from build123d import *

# Parameters (mm, degrees)
SKETCH_2_W          = 460
SKETCH_2_H          = 110
EXTRUDE_1_DEPTH     = 8
SKETCH_4_R          = 1.5
CUT_EXTRUDE_1_DEPTH = 237.619948441
SKETCH_3_R          = 2.5
SKETCH_3_R_2        = 1.5
CUT_EXTRUDE_2_DEPTH = 237.619948441
FILLET_1_R          = 10


with BuildPart() as part:
    # 草图2 → 凸台-拉伸1 (new body)
    with BuildSketch(Plane(origin=(0, 0, 0), x_dir=(1, 0, 0), z_dir=(0, 1, 0))):
        Rectangle(SKETCH_2_W, SKETCH_2_H)
    extrude(amount=EXTRUDE_1_DEPTH)

    # 草图4 → 切除-拉伸1 (cut, through all)
    with BuildSketch(Plane(origin=(0, 8, 0), x_dir=(1, 0, 0), z_dir=(0, 1, 0))):
        with Locations(Location((-70, 35, 0), (0, 0, 270))):
            Circle(SKETCH_4_R)
        with Locations(Location((-70, -43, 0), (0, 0, 270))):
            Circle(SKETCH_4_R)
        with Locations(Location((-215, -43, 0), (0, 0, 270))):
            Circle(SKETCH_4_R)
        with Locations(Location((-215, 40, 0), (0, 0, 270))):
            Circle(SKETCH_4_R)
        with Locations(Location((-170, -43, 0), (0, 0, 270))):
            Circle(SKETCH_4_R)
        with Locations(Location((-215, -1.5, 0), (0, 0, 270))):
            Circle(SKETCH_4_R)
    cut_extrude_1 = extrude(amount=-CUT_EXTRUDE_1_DEPTH, mode=Mode.SUBTRACT)

    # 草图3 → 切除-拉伸2 (cut, through all)
    with BuildSketch(Plane(origin=(0, 8, 0), x_dir=(1, 0, 0), z_dir=(0, 1, 0))):
        with Locations(Location((-120, 25, 0), (0, 0, 270))):
            Circle(SKETCH_3_R)
        with Locations(Location((-120, -5, 0), (0, 0, 270))):
            Circle(SKETCH_3_R)
        with Locations(Location((-152, 32.5, 0), (0, 0, 270))):
            Circle(SKETCH_3_R_2)
        with Locations(Location((-152, 22.5, 0), (0, 0, 270))):
            Circle(SKETCH_3_R_2)
        with Locations(Location((-96, 32.5, 0), (0, 0, 270))):
            Circle(SKETCH_3_R_2)
        with Locations(Location((-96, 22.5, 0), (0, 0, 270))):
            Circle(SKETCH_3_R_2)
        Polygon((-70, 55), (-48.5526258, 35), (48.5526258, 35), (70, 55), align=None)
    cut_extrude_2 = extrude(amount=-CUT_EXTRUDE_2_DEPTH, mode=Mode.SUBTRACT)

    # 镜向1: 切除-拉伸1, 切除-拉伸2 across plane
    add(cut_extrude_1.mirror(Plane(origin=(0, 0, 0), x_dir=(0, 0, 1), z_dir=(1, 0, 0))), mode=Mode.SUBTRACT)
    add(cut_extrude_2.mirror(Plane(origin=(0, 0, 0), x_dir=(0, 0, 1), z_dir=(1, 0, 0))), mode=Mode.SUBTRACT)

    # 圆角1
    fillet_1_edges = [part.edges().sort_by_distance(p)[0] for p in [
        (-70, 4, -55),
        (70, 4, -55),
        (48.5526258, 4, -35),
        (-48.5526258, 4, -35),
        (-230, 4, -55),
        (230, 4, -55),
    ]]
    fillet(fillet_1_edges, radius=FILLET_1_R)


solid = part.part
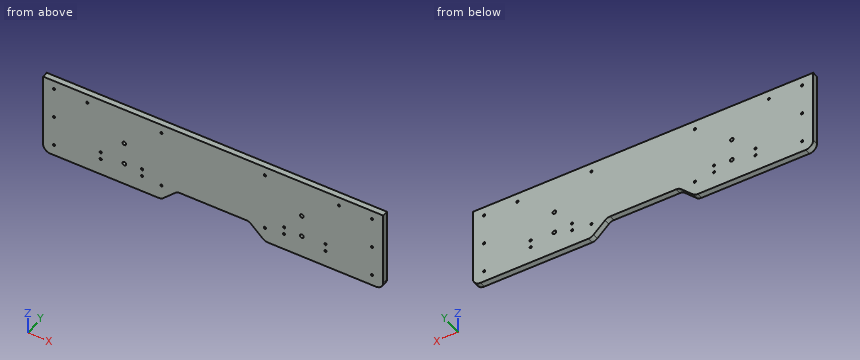
Can you work these out from the model? Positions are in its coordinate system, mm. Give positions to 0.01 mm unless a question says otherwise; leave off trailing zeros. Order: outer loops, then holes, each group sorted by start corner. A loop starts at its lowest first (then second) coordinate and runs counter-clockwise, first axis right, second up. Notation, with made-up numbers: M -6,64 L 18,64 A19 ccw 18,83 Z; hole C 11.5,83.5 d3. An arc over 180 degrees is marked long. One line per item, written item: value.
Item 1: If we section it at A-A on y = 4.75: State how many separate pieces and enclosed holes the cut face has, and give its area (3 significant figures).
Verdict:
separate pieces: 1
enclosed holes: 24
area: 48,000 mm2
Item 2: If we section it at B-B on x = -33: Write out the boundary of the cut face in (y, z), and give its area (3 significant figures).
Verdict:
outline: M 0,-35 L 8,-35 L 8,55 L 0,55 Z
area: 720 mm2
Item 3: Please list where these lines run through material, in increasing order: line 1 (X direction, y = 5.75, z = 5); line 2 (Z direction, x = -152, y = 5); line 3 (X direction, y = 2, z = -32.5).
Verdict:
line 1: -230 to -122.5, -117.5 to 117.5, 122.5 to 230
line 2: -55 to -34, -31 to -24, -21 to 55
line 3: -230 to -153.5, -150.5 to -97.5, -94.5 to 94.5, 97.5 to 150.5, 153.5 to 230
